Can you work these out from the drawing? Everything is in mm from the part's minimum corner. A direction names the side the tool comes from. Give positions to 0.01 mm unless a question says otherwise; leave off trailing zeros. Loops run counter-clockwise (first coordinate to the right, second up) from the corner with the lowest first, then second, coordinate; pieces in that order, holes last. Notation, with made-up numbers: (-28, -29.5) -> (22, -29.5) arc R17 cw to (22, -3.5) -> close; hole circle Ø2 at (63.25, 74). An arc over 180 degrees is marked (long way). Write item = value, one per line. Start each with the question number.
1) I want a section at B-B (x = 15). List the corners of the cut face in (y, z) for me.
2) I'm going to push flat-ended pins straight in: pin 1 Ø2.5 at (y, z) = (15.69, 24) entering from +X; pin 2 Ø4 at (x, z) = (15, 25) entering from +Y. Where does each tip first touch, or does it pass through?
3) On a 3-axis mill with a long thin cutter (end or side, diameter ignored), from which of +Z, -Z, +X, -X, +Y, -Y can I reach the whole of each face in a straight line? I mean the marked faces 1 and 2. Say none if no direction works.
4) I want a section at A-A (y = 33.5). List the corners of the cut face in (x, z) for me, and give its area (3 significant figures).
5) I want a section at D-D (y = 6). List the corners of the cut face in (x, z) for me.
6) I need wall thicknesses on probe 1 along X at (y, z) = (36, 2.75); probe 2 along Z at (x, y) = (15, 1.6); probe 3 along Y at (x, z) = (29.25, 24). Which ranges of each line are inside material? Lowest first, please. Write a range as from..to.
7) I want a section at C-C (z = 5). List the corners of the cut face in (x, y) for me.
8) If we mould it in two halves opening along X, with no side actions, what happens to the marked faces 3, 4 and 5? For each: +X half, -X half, draft (parallel to the pull), parting line (faces both ways), or undercut.
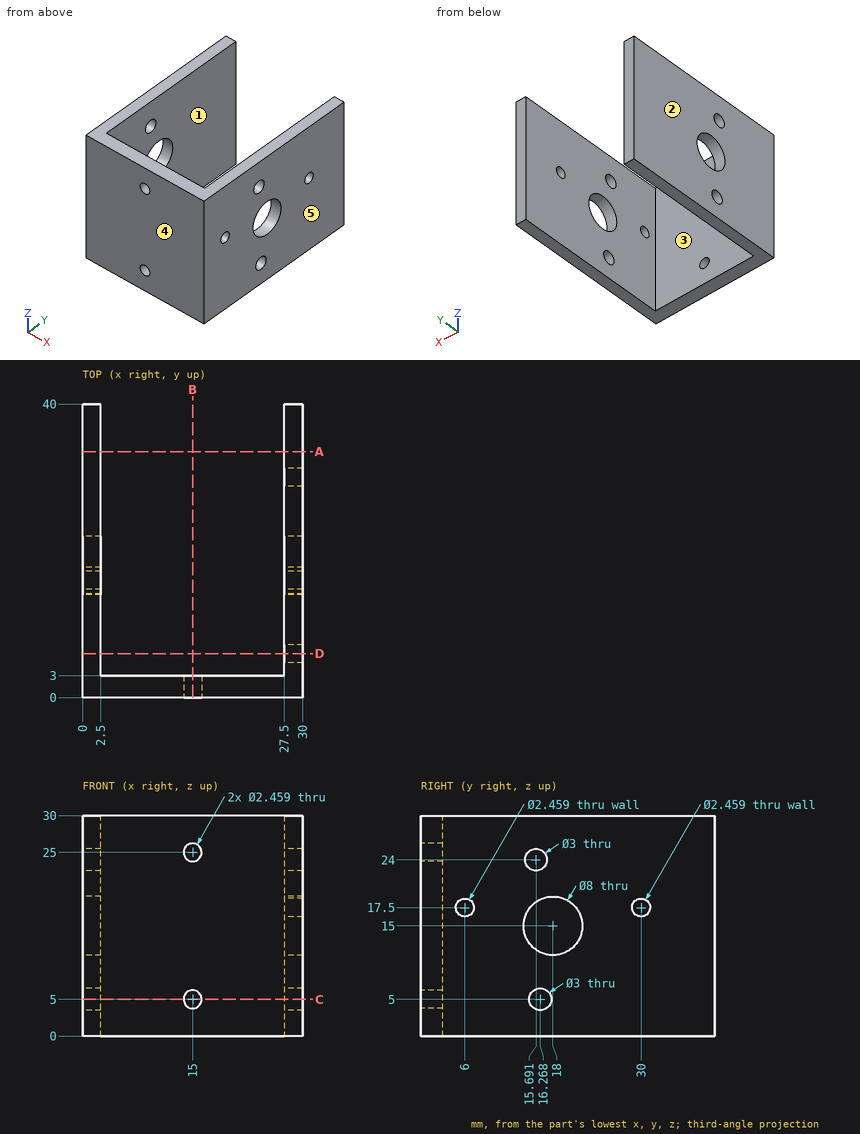
Answer list:
q1.outline = (0, 0) -> (3, 0) -> (3, 3.77) -> (0, 3.77) -> close; (0, 6.23) -> (3, 6.23) -> (3, 23.77) -> (0, 23.77) -> close; (0, 26.23) -> (3, 26.23) -> (3, 30) -> (0, 30) -> close
q2.pin_1 = through
q2.pin_2 = 3
q3.face_1 = +Z, -Z, +Y
q3.face_2 = +Z, -Z, -X, +Y, -Y
q4.outline = (0, 0) -> (2.5, 0) -> (2.5, 30) -> (0, 30) -> close; (27.5, 0) -> (30, 0) -> (30, 30) -> (27.5, 30) -> close
q4.area = 150 mm^2
q5.outline = (0, 0) -> (2.5, 0) -> (2.5, 30) -> (0, 30) -> close; (27.5, 0) -> (30, 0) -> (30, 16.27) -> (27.5, 16.27) -> close; (27.5, 18.73) -> (30, 18.73) -> (30, 30) -> (27.5, 30) -> close
q6.probe_1 = 0..2.5, 27.5..30
q6.probe_2 = 0..3.77, 6.23..23.77, 26.23..30
q6.probe_3 = 0..14.19, 17.19..40
q7.outline = (0, 0) -> (13.77, 0) -> (13.77, 3) -> (2.5, 3) -> (2.5, 14.77) -> (0, 14.77) -> close; (0, 17.77) -> (2.5, 17.77) -> (2.5, 40) -> (0, 40) -> close; (16.23, 0) -> (30, 0) -> (30, 14.77) -> (27.5, 14.77) -> (27.5, 3) -> (16.23, 3) -> close; (27.5, 17.77) -> (30, 17.77) -> (30, 40) -> (27.5, 40) -> close
q8.face_3 = undercut
q8.face_4 = draft
q8.face_5 = +X half
